Autodesk Inventor part; units mm, degrees
ref_plane "YZ Plane" through (0, 0, 0) normal (1, 0, 0) x (0, 1, 0)
ref_plane "XZ Plane" through (0, 0, 0) normal (0, 1, 0) x (-1, 0, 0)
ref_plane "XY Plane" through (0, 0, 0) normal (0, 0, 1) x (1, 0, 0)
sketch "Sketch1" plane through (0, 0, 0) normal (0, 1, 0) x (-1, 0, 0)
  line L0 (0, 0) -> (20, 0)
  line L1 (20, 0) -> (20, -50)
  line L2 (20, -50) -> (0, -50)
  line L3 (0, -50) -> (0, 0)
  dimension "d0" = 50
  dimension "d1" = 20
extrude "Extrusion1" add sketch "Sketch1" along normal blind 10
sketch "Sketch4" plane through (0, 10, 0) normal (0, 1, 0) x (1, 0, 0)
  line L0 (-18.73, 16.39) -> (-18.73, 11.39)
  line L1 (-18.73, 11.39) -> (-8.73, 11.39)
  line L2 (-8.73, 11.39) -> (-8.73, 6.39) construction
  line L3 (-18.73, 16.39) -> (-8.73, 16.39)
  arc A0 (-8.73, 6.39) -> (-8.73, 11.39) centre (-8.73, 8.89) ccw
  line L4 (-8.73, 6.39) -> (-8.73, 1.39)
  arc A1 (-15.8011, 11.39) -> (-8.73, 1.39) centre (-8.73, 8.89) ccw construction
  line L5 (-20, 0) -> (0, 0) construction
  line L6 (0, 0) -> (0, 50) construction
  line L7 (0, 50) -> (-20, 50) construction
  line L8 (-20, 50) -> (-20, 0) construction
  line L9 (-20, 0) -> (0, 0)
  line L10 (-10, 0) -> (-10, 50) construction
  arc A2 (-10, 16.2817) -> (-15.8011, 11.39) centre (-8.73, 8.89) ccw construction
  arc A3 (-8.73, 1.39) -> (-10, 16.2817) centre (-8.73, 8.89) ccw
  arc A4 (-10, 6.7366) -> (-8.73, 6.39) centre (-8.73, 8.89) ccw construction
  arc A5 (-8.73, 11.39) -> (-10, 6.7366) centre (-8.73, 8.89) ccw construction
  line L11 (-1.23, 8.89) -> (-1.23, 50) construction
  line L12 (-1.23, 16.7009) -> (-18.73, 21.39)
  line L13 (-18.73, 21.39) -> (-18.73, 26.39)
  line L14 (-18.73, 26.39) -> (-1.23, 31.0791)
  line L15 (-1.23, 32.39) -> (-18.73, 32.39)
  line L16 (-1.23, 16.7009) -> (-1.23, 21.7009)
  line L17 (-6.23, 22.64) -> (-1.23, 21.7009)
  line L18 (-6.23, 22.64) -> (-6.23, 25.14)
  line L19 (-6.23, 25.14) -> (-1.23, 26.0791)
  line L20 (-1.23, 31.0791) -> (-1.23, 26.0791)
  line L21 (-18.73, 23.89) -> (-1.23, 23.89) construction
  line L22 (-14.98, 23.89) -> (-9.98, 22.5503)
  line L23 (-9.98, 22.5503) -> (-9.98, 25.2297)
  line L24 (-9.98, 25.2297) -> (-14.98, 23.89)
  line L25 (-1.23, 32.39) -> (-1.23, 42.39)
  line L26 (-1.23, 42.39) -> (-9.375, 42.39)
  line L27 (-10, 42.39) -> (-10, 42.39)
  line L28 (-10, 42.39) -> (-10.625, 42.39)
  line L29 (-18.73, 42.39) -> (-18.73, 32.39)
  line L30 (-8.73, 35.64) -> (-3.73, 35.64)
  line L31 (-3.73, 35.64) -> (-3.73, 39.14)
  line L32 (-3.73, 39.14) -> (-8.73, 39.14)
  line L33 (-8.73, 39.14) -> (-8.73, 35.64)
  line L34 (-6.23, 32.39) -> (-6.23, 42.39) construction
  line L35 (-6.23, 37.39) -> (-1.23, 37.39) construction
  line L36 (-6.23, 37.39) -> (-10, 37.39) construction
  line L37 (-15.23, 35.64) -> (-12.23, 35.64)
  line L38 (-12.23, 35.64) -> (-12.23, 39.14)
  line L39 (-12.23, 39.14) -> (-15.23, 39.14)
  line L40 (-15.23, 39.14) -> (-15.23, 35.64)
  line L41 (-12.23, 37.39) -> (-10, 37.39) construction
  line L42 (-20, 50) -> (-20, 0)
  line L43 (-20, 0) -> (-20, 50)
  line L44 (0, 50) -> (-20, 50)
  line L45 (-20, 50) -> (0, 50)
  line L46 (0, 50) -> (0, 0)
  line L47 (-10.625, 42.39) -> (-10, 41.14)
  line L48 (-10, 41.14) -> (-9.375, 42.39)
  line L49 (-10, 42.39) -> (-10.625, 42.39)
  line L50 (-10, 42.39) -> (-9.375, 42.39)
  line L51 (-10.625, 42.39) -> (-18.73, 42.39)
  line L52 (-9.375, 42.39) -> (-10, 42.39)
  point P0 (-6.23, 23.89)
  point P1 (-9.98, 23.89)
  point P2 (-6.23, 39.14)
  point P3 (-8.73, 37.39)
  dimension "d11" = 5
  dimension "d12" = 10
  dimension "d14" = 5
  dimension "d16" = 10
  dimension "d17" = 1.27
  dimension "d18" = 8.89
  dimension "d19" = 75
  dimension "d20" = 75
  dimension "d21" = 5
  dimension "d22" = 2.5
  dimension "d23" = 15
  dimension "d24" = 5
  dimension "d25" = 5
  dimension "d26" = 8.5
  dimension "d27" = 10
  dimension "d28" = 10
  dimension "d29" = 5
  dimension "d34" = 3.5
  dimension "d35" = 1.25
  dimension "d36" = 1.25
  dimension "d39" = 2.5
  dimension "d40" = 3.5
  dimension "d41" = 3.5
extrude "Extrusion3" cut sketch "Sketch4" against normal blind 5 contours L42 L44 L46 L9 | L48 L47 L28 L50 | L24 L23 L22 | L33 L32 L31 L30 | L40 L39 L38 L37
fillet "Fillet1" radius 3.175 4 edges at (-18.73, 7.5, -42.39) (-10.625, 7.5, -42.39) (-9.375, 7.5, -42.39) (-1.23, 7.5, -42.39)
sketch "Sketch5" plane through (0, 5, 0) normal (0, 1, 0) x (1, 0, 0)
  line L0 (-20, 50) -> (0, 50)
  line L1 (-20, 0) -> (-20, 50)
  line L2 (0, 0) -> (-20, 0)
  point P0 (-15, 5)
  point P1 (-15, 46.5)
  dimension "d43" = 3.5
  dimension "d44" = 5
  dimension "d45" = 5
  dimension "d46" = 5
hole "Hole1" at (-15, 5, -5) at (-15, 5, -46.5) direction (0, -1, 0) diameter 3.175 end through all counterbore diameter 5.08 counterbore depth 2.54
fillet "Fillet2" radius 0.9525 4 edges at (-8.73, 7.5, -39.14) (-3.73, 7.5, -39.14) (-12.23, 7.5, -39.14) (-15.23, 7.5, -39.14)
equation "\"d20\" = d19"
equation "\"d22\" = 0.5 * d21"
properties part number "initials"
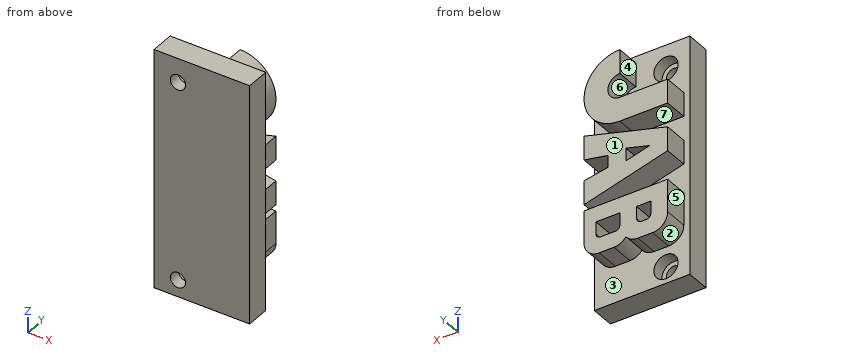
Could you check a few things on this model? Use its own coordinates, in mm. Face numbers are marked on the shaded views. A direction names the side the tool comes from. Give positions to 0.01 mm unless a question says otherwise; leave off trailing zeros. Write each loop counter-clockwise with the first axis right and the second up, starting at its lowest first coordinate (ties: lowest second). Pieces come first, ordered by that corner, then holes. Notation, with made-up numbers: (53.5, -4) -> (61.5, -4) arc R35 ccw to (61.5, 30) -> close; hole circle Ø6 at (83.5, -30.5). An arc over 180 degrees is marked (long way). Write each question's results on one line, items separated by ' | '.
1. If we mould it in two halves opening along Z, with no side actions, what happens to the marked faces 1, 2 and 3? For each: released by +Z, released by -Z, zero draft, split by the parting line, or undercut.
Check sheet entries:
face 1: zero draft | face 2: released by -Z | face 3: undercut
2. I want a section at A-A, the plane z = -46.5. Write out the boundary of the cut face in (x, y).
Check sheet entries:
outline: (-20, 0) -> (-16.59, 0) -> (-16.59, 2.46) -> (-17.54, 2.46) -> (-17.54, 5) -> (-20, 5) -> close; (-13.41, 0) -> (0, 0) -> (0, 5) -> (-12.46, 5) -> (-12.46, 2.46) -> (-13.41, 2.46) -> close
3. I need wall thicknesses on L1, parallel to Z at x = -15, y = 4.15; L2, parallel to X at y = 8.5, z = -38; L3, parallel to Z at x = -15, y = 2. Which ranges of each line are inside material? Lowest first, please.
Check sheet entries:
L1: z = -50 to -49.04, -43.96 to -7.54, -2.46 to 0 | L2: x = -18.73 to -15.23, -12.23 to -8.73, -3.73 to -1.23 | L3: z = -50 to -48.09, -44.91 to -6.59, -3.41 to 0
4. On a 3-axis mill with a long thin cutter (end or side, diameter ignored), from which of +Z, -Z, +X, -X, +Y, -Y can I reach the whole of each face in a straight line? I mean the marked faces 4, 5, 6 and 7. Say none if no direction works.
Check sheet entries:
face 4: +Z, -X, +Y | face 5: +Z, -Z, -X, +Y | face 6: -X, +Y | face 7: +X, -X, +Y
5. Will these pins go through, and if not, where does the flat tip stop? pin 1 Ø0.9 at (x, y) = (-13.5, 8) entering from +Z; pin 2 Ø1.8 at (x, z) = (-7.5, -36.5) entering from +Y; pin 3 Ø2.5 at (y, z) = (8, -25) entering from -X; pin 4 Ø1.5 at (y, z) = (7, -9) entering from +X.
Check sheet entries:
pin 1: stops at z = -11.39 | pin 2: stops at y = 10 | pin 3: stops at x = -18.73 | pin 4: stops at x = -1.23
6. I want a section at D-D, the plane y = 7.5. Count the separate pieces of the cut face and the enclosed holes in it, then the cut area to 3 significant figures.
Check sheet entries:
separate pieces: 3 | enclosed holes: 3 | area: 416 mm²
7. I want a section at B-B, the plane z = -34.5. Write out the boundary of the cut face in (x, y), then the cut area to 4 significant figures.
Check sheet entries:
outline: (-20, 0) -> (0, 0) -> (0, 5) -> (-1.23, 5) -> (-1.23, 10) -> (-18.73, 10) -> (-18.73, 5) -> (-20, 5) -> close | area: 187.5 mm²
8. I want a section at C-C, the plane y = 2. Write out the boundary of the cut face in (x, z) (1 decimal), then the cut area to 3 significant figures.
Check sheet entries:
outline: (-20, -50) -> (0, -50) -> (0, 0) -> (-20, 0) -> close; hole circle Ø3.2 at (-15, -46.5); hole circle Ø3.2 at (-15, -5) | area: 984 mm²
